The listing builds one solid part. Answer for the finished solid, in the listing's coordinates (mm). A direction names the side the tool comes from. Give positions to 0.01 mm unless a question says otherwise; leave off trailing zeros. Write each loop counter-clockwise with the first axis right and the second up, starting at its lowest first coordinate (ties: lowest second). Pieces come first, ordered by that corner, then holes. Notation, with made-up numbers: (15.5, -21) - (56.5, -21) arc R12 ccw to (56.5, -16) - close; hole circle Ø6 at (-31, 40). An arc over 180 degrees is marked (long way). One line per item, written item: value. Start each with the question number.
from build123d import *

# Parameters (mm, degrees)
F0_R           = 19.0832795918
F1_DEPTH       = 25.4
F2_D           = 6.6
F3_W           = 11.2244253978
F3_H           = 9.497590363
F4_DEPTH       = 50.8
F6_D           = 6.6
F7_D           = 6.6
F7_CBORE_D     = 11.25
F7_CBORE_DEPTH = 6


with BuildPart() as f1:
    # F0 (on Front) → F1 (new body)
    with BuildSketch(Plane.XZ):
        Circle(F0_R)
    extrude(amount=F1_DEPTH)

    # F2 (through all)
    with Locations(Plane(origin=(0, 0, 0), x_dir=(1, 0, 0), z_dir=(0, 1, 0))):
        with Locations((0, -12.8073552623), (12.8073552623, 0), (0, 12.8073552623), (-12.8073552623, 0)):
            Hole(F2_D / 2)

    # F3 (on face) → F4 (join)
    with BuildSketch(Plane.XZ.offset(25.4)):
        Rectangle(F3_W, F3_H)
    extrude(amount=F4_DEPTH)

    # F6 (through all)
    with Locations(Plane(origin=(0, 0, -4.7487951815), x_dir=(1, 0, 0), z_dir=(0, 0, -1))):
        with Locations((0, 44.753793627)):
            Hole(F6_D / 2)

    # F7 (through all)
    with Locations(Plane(origin=(0, 0, 0), x_dir=(1, 0, 0), z_dir=(0, 1, 0))):
        with Locations((0, 0)):
            CounterBoreHole(F7_D / 2, F7_CBORE_D / 2, F7_CBORE_DEPTH)


solid = f1.part
Item 1: For faces 4 (the cylindrical face through (2.6, -2.96, 4.99)), 5 (the flat face through (0, -50, -4.749)), 6 (the flat face through (0, -50, 4.749)), 7 (the flat face through (-5.612, -50, 0)), determine the directions among +Z, -Z, +X, -X, +Y, -Y from which every point of the face is accessible in a straight line to the end or side of a thin tool.
Item 2: Find section C-C on x = -14. Determine the outline of the cut face in (y, z), plus the area to 3 significant figures.
Item 3: The mould has two halves that part along Z. Classify faces 1 (the flat face through (-3, -76.2, 2)), 2 (the cylindrical face through (-10.375, -12.878, -2.23)), 3 (the cylindrical face through (-4.14, -12.52, -18.63)): +Z half, -Z half, draft (parallel to the pull), parting line (faces both ways), or undercut.
Item 4: Find section B-B on y = -61. Determine the outline of the cut face in (x, z), plus the area to 3 significant figures.
Item 5: Find section A-A on x = 0. Give the number of separate pieces and of enclosed holes in the cut face, plus the area to 3 significant figures.
Item 6: Each of these flat-tipped pins is pushed along its axis until it touches: pin 1 Ø8 at (x, y) = (-4.5, -27.5) entering from -Z; pin 2 Ø12.5 at (x, y) = (1.5, -48.5) entering from +Z; pin 3 Ø10.5 at (y, z) = (-39, -2.5) entering from -X. Where does it stop, or does it pass through?
Item 7: Straight lines are drawn through the part: line 1 along Z through (x, y) = (0, -18); line 2 along Z through (x, y) = (0, -54); line 3 along Z through (x, y) = (0, -5.75) (3 decimals). For each, find the intervals that lie inside material, in ascending order.
Item 8: Find section D-D on z = -10.5. Determine the outline of the cut face in (x, y), plus the area to 3 significant figures.
Values:
1. face 4: +Y
1. face 5: -Z, +X, -X, -Y
1. face 6: +Z, +X, -X, -Y
1. face 7: +Z, -Z, -X, -Y
2. outline: (-25.4, -12.97) - (0, -12.97) - (0, -3.08) - (-25.4, -3.08) - close; (-25.4, 3.08) - (0, 3.08) - (0, 12.97) - (-25.4, 12.97) - close
2. area: 502 mm^2
3. face 1: draft
3. face 2: undercut
3. face 3: parting line
4. outline: (-5.61, -4.75) - (5.61, -4.75) - (5.61, 4.75) - (-5.61, 4.75) - close; hole circle Ø6.6 at (0, 0)
4. area: 72.4 mm^2
5. separate pieces: 6
5. enclosed holes: 0
5. area: 567 mm^2
6. pin 1: z = -19.05
6. pin 2: z = 4.75
6. pin 3: x = -5.61
7. line 1: -19.08 to -16.11, -9.51 to -3.3, 3.3 to 9.51, 16.11 to 19.08
7. line 2: -4.75 to -3.3, 3.3 to 4.75
7. line 3: -19.083 to -16.107, -9.507 to -5.625, 5.625 to 9.507, 16.107 to 19.083
8. outline: (-15.93, -25.4) - (-2.36, -25.4) - (-2.36, 0) - (-15.93, 0) - close; (2.36, -25.4) - (15.93, -25.4) - (15.93, 0) - (2.36, 0) - close
8. area: 690 mm^2
